Autodesk Inventor part; units mm, degrees
ref_plane "YZ Plane" through (0, 0, 0) normal (1, 0, 0) x (0, 1, 0)
ref_plane "XZ Plane" through (0, 0, 0) normal (0, 1, 0) x (-1, 0, 0)
ref_plane "XY Plane" through (0, 0, 0) normal (0, 0, 1) x (1, 0, 0)
sketch "Sketch1" plane through (0, 0, 0) normal (0, 0, 1) x (1, 0, 0)
  line L0 (-25, 20) -> (25, 20)
  line L1 (25, 20) -> (25, -20)
  line L2 (25, -20) -> (-25, -20)
  line L3 (-25, -20) -> (-25, 20)
  point P0 (0, 0)
  point P1 (0, 20)
  point P2 (-25, 0)
  dimension "d0" = 50
  dimension "d1" = 40
extrude "Extrusion1" add sketch "Sketch1" along normal blind 8
sketch "Sketch5" plane through (0, 0, 0) normal (0, 0, -1) x (-1, 0, 0)
  circle A0 centre (-15.5, -16.5) radius 1
  circle A1 centre (15.5, -16.5) radius 1
  circle A2 centre (-15.5, 14.5) radius 1
  circle A3 centre (15.5, 14.5) radius 1.25
  arc A4 (-2, -2.5) -> (-2, 0.5) centre (0, -1) ccw
  line L0 (-2, -2.5) -> (-2, 0.5)
  circle A5 centre (0, -1) radius 4
  point P0 (0, 0)
  dimension "d29" = 8
extrude "Extrusion5" cut sketch "Sketch5" against normal through all contours A0 | A1 | A2 | A3 | L0 A4 | A5
properties part number "0005-10-020 suport motor y"
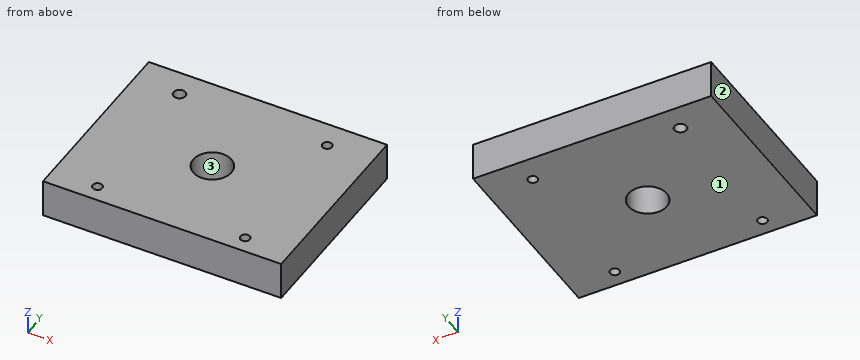
Can you work these out from the model? Positions are in its coordinate system, mm. Face numbers are marked on the shaded views. Coordinates: 2 decimals unless noted, no trailing zeros. Loops run counter-clockwise (first coordinate to the right, second up) from the corner with the lowest first, then second, coordinate; pieces in that order, holes last.
1) Imagine slicing it at C-C on x = 0. List the corners of the cut face in (y, z) for me.
2) Imagine slicing it at B-B on y = -1. List the corners of the cut face in (x, z) for me, plus the area to 3 significant figures.
3) Imagine slicing it at A-A on x = 15.5. List the corners of the cut face in (y, z) for me.
4) Imagine slicing it at D-D on z = 3.75. List the corners of the cut face in (x, y) for me.
5) I need wall thicknesses on probe 1 along Y at (x, z) = (-15.5, 4); probe 2 along Y at (x, z) = (0, 5.25); probe 3 along Y at (x, z) = (15.5, 5.25). Which ranges of each line are inside material? Lowest first, please.
6) Thinking about a two-plate mould opening in X: for the marked faces 1, 2 and 3, which applies, pulls with the +X half, pulls with the -X half, needs draft (parallel to the pull), parting line crosses it, or undercut?
Completed:
1. outline: (-20, 0) - (-5, 0) - (-5, 8) - (-20, 8) - close; (3, 0) - (20, 0) - (20, 8) - (3, 8) - close
2. outline: (-25, 0) - (-4, 0) - (-4, 8) - (-25, 8) - close; (4, 0) - (25, 0) - (25, 8) - (4, 8) - close
2. area: 336 mm2
3. outline: (-20, 0) - (-17.5, 0) - (-17.5, 8) - (-20, 8) - close; (-15.5, 0) - (13.5, 0) - (13.5, 8) - (-15.5, 8) - close; (15.5, 0) - (20, 0) - (20, 8) - (15.5, 8) - close
4. outline: (-25, -20) - (25, -20) - (25, 20) - (-25, 20) - close; hole circle Ø2.5 at (-15.5, 14.5); hole circle Ø2 at (-15.5, -16.5); hole circle Ø8 at (0, -1); hole circle Ø2 at (15.5, -16.5); hole circle Ø2 at (15.5, 14.5)
5. probe 1: y = -20 to -17.5, -15.5 to 13.25, 15.75 to 20
5. probe 2: y = -20 to -5, 3 to 20
5. probe 3: y = -20 to -17.5, -15.5 to 13.5, 15.5 to 20
6. face 1: needs draft
6. face 2: pulls with the -X half
6. face 3: undercut
